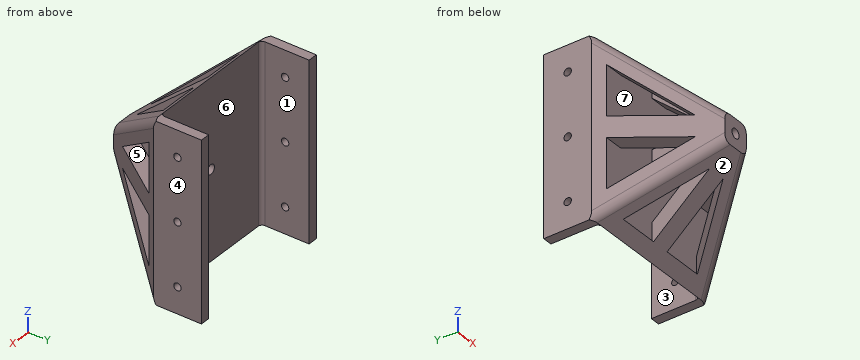
from build123d import *

# Parameters (mm, degrees)
BOSS_EXTRUDE1_DEPTH = 117.094
SKETCH3_R           = 2.4384
CUT_EXTRUDE1_DEPTH  = 166.226170252
SKETCH4_R           = 3.175
CUT_EXTRUDE2_DEPTH  = 166.226170252
CUT_EXTRUDE3_DEPTH  = 166.226170252
FILLET1_R           = 6.35
CUT_EXTRUDE4_DEPTH  = 166.226170252
CUT_EXTRUDE5_DEPTH  = 110.744


with BuildPart() as part:
    # Sketch2 → Boss-Extrude1 (new body)
    with BuildSketch(Plane.XY):
        with BuildLine():
            Line((95.25, 31.75), (101.6, 31.75))
            Line((101.6, 31.75), (101.6, 0))
            Line((101.6, 0), (60.325, -57.15))
            Line((60.325, -57.15), (41.275, -57.15))
            Line((41.275, -57.15), (0, 0))
            Line((0, 0), (0, 31.75))
            Line((0, 31.75), (6.35, 31.75))
            Line((6.35, 31.75), (6.35, 2.54))
            ThreePointArc((6.35, 2.54), (7.093948776, 0.743948776), (8.89, 0))
            Line((8.89, 0), (92.71, 0))
            ThreePointArc((92.71, 0), (94.506051224, 0.743948776), (95.25, 2.54))
            Line((95.25, 2.54), (95.25, 31.75))
        make_face()
    extrude(amount=BOSS_EXTRUDE1_DEPTH)

    # Sketch3 → Cut-Extrude1 (cut, through all)
    with BuildSketch(Plane(origin=(101.6, 0, 0), x_dir=(0, 0, -1), z_dir=(1, 0, 0))):
        with Locations((-99.822, 15.875)):
            Circle(SKETCH3_R)
        with Locations((-58.547, 15.875)):
            Circle(SKETCH3_R)
        with Locations((-17.272, 15.875)):
            Circle(SKETCH3_R)
    extrude(amount=-CUT_EXTRUDE1_DEPTH, mode=Mode.SUBTRACT)

    # Sketch4 → Cut-Extrude2 (cut, through all)
    with BuildSketch(Plane(origin=(0, 0, 0), x_dir=(1, 0, 0), z_dir=(0, 1, 0))):
        with Locations(Location((50.8, -58.547, 0), (0, 0, 270))):
            Circle(SKETCH4_R)
    extrude(amount=-CUT_EXTRUDE2_DEPTH, mode=Mode.SUBTRACT)

    # Sketch5 → Cut-Extrude3 (cut, through all)
    with BuildSketch(Plane(origin=(101.6, 0, 0), x_dir=(0, 0, -1), z_dir=(1, 0, 0))):
        Polygon((-117.094, 0), (-117.094, -57.15), (-68.072, -57.15), align=None)
        Polygon((-49.022, -57.15), (0, -57.15), (0, 0), align=None)
    extrude(amount=-CUT_EXTRUDE3_DEPTH, mode=Mode.SUBTRACT)

    # Fillet1
    fillet1_edges = [part.edges().sort_by_distance(p)[0] for p in [
        (80.9625, -28.575, 92.583),
        (20.6375, -28.575, 92.583),
        (80.9625, -28.575, 24.511),
        (20.6375, -28.575, 24.511),
    ]]
    fillet(fillet1_edges, radius=FILLET1_R)

    # Sketch7 → Cut-Extrude4 (cut, through all)
    with BuildSketch(Plane(origin=(101.6, 0, 0), x_dir=(0, 0, -1), z_dir=(1, 0, 0))):
        Polygon((-98.104076531, -6.35), (-65.422743198, -44.45), (-65.422743198, -6.35), align=None)
        Polygon((-18.989923469, -6.35), (-51.671256802, -6.35), (-51.671256802, -44.45), align=None)
    extrude(amount=-CUT_EXTRUDE4_DEPTH, mode=Mode.SUBTRACT)

    # Sketch8 → Cut-Extrude5 (cut)
    with BuildSketch(Plane.XY.offset(117.094)):
        Polygon((17.266111361, -6.35), (44.782778028, -44.45), (44.782778028, -6.35), align=None)
        Polygon((84.333888639, -6.35), (56.817221972, -6.35), (56.817221972, -44.45), align=None)
    extrude(amount=-CUT_EXTRUDE5_DEPTH, mode=Mode.SUBTRACT)


solid = part.part
Part model, mm, in its own coordinate system. Face numbers are marked on the shaded views. A direction names the side the tool comes from. Coordinates: 2 decimals unless noted, no trailing zeros. Write each loop counter-clockwise with the first axis right and the second up, starting at its lowest first coordinate (ties: lowest second). Pieces come first, ordered by that corner, then holes. Notation, with made-up numbers: (-2, -29) - (44, -29) arc R13 cw to (44, -15) - close; hole circle Ø10 at (34.25, 56.25). An arc over 180 degrees is marked (long way). Put each result on its own line as item: value.
1. 3-axis set-ups, long thin cutter, end or side, ignore diameter. For the marked faces 5, 6 and 7: which of +Z, -Z, +X, -X, +Y, -Y reach the whole face in a straight line?
Final values:
face 5: +X, -X
face 6: +Z, -Z, +Y
face 7: none
2. Two-plate mould, pull along X, no slides. Class the marked faces 1, 2, 3 and 4: +X half, -X half, draft (parallel to the pull), parting line (faces both ways), or undercut.
Final values:
face 1: undercut
face 2: draft
face 3: undercut
face 4: +X half
3. Probe line 1 along X through (y, z) = (12, 25.5); line 2 along Z through (x, y) = (50.5, -39); line 3 along X through (y, z) = (-36, 41.5). List the from-to ranges inside material, lowest first. Write a range as [from, to].
Final values:
line 1: x = [0, 6.35], [95.25, 101.6]
line 2: z = [33.45, 47], [51.67, 55.39], [61.71, 65.42], [70.1, 83.64]
line 3: x = [26, 38.68], [44.78, 56.82], [62.92, 75.6]
4. Band-saw the part on B-B (x = 50.8). Write the cut outline in (y, z).
Final values:
outline: (-57.15, 49.02) - (0, 0) - (0, 55.37) - (-57.15, 55.37) - close; (-57.15, 61.72) - (0, 61.72) - (0, 117.09) - (-57.15, 68.07) - close; hole (-44.45, 51.67) - (-6.35, 18.99) - (-6.35, 51.67) - close; hole (-44.45, 65.42) - (-6.35, 65.42) - (-6.35, 98.1) - close
5. Band-saw the part on C-C (z = 27). Give the number of separate pieces and of enclosed holes in the cut face, then the cut area to 3 significant figures.
Final values:
separate pieces: 4
enclosed holes: 0
area: 1,600 mm²
6. Flat gauge pins, fed straight in: pin 1 Ø4 at (y, z) = (15.875, 17.272) entering from +X; pin 2 Ø11.5 at (y, z) = (-17.5, 24.5) entering from +X; pin 3 Ø5 at (x, z) = (30, 46.5) entering from +Y; pin 4 Ø9.5 at (x, y) = (51, -28) entering from -Z. Where does each tip first touch, or does it go through?
Final values:
pin 1: passes through
pin 2: stops at x = 93.07
pin 3: stops at y = 0
pin 4: stops at z = 19.94
7. Band-saw the part on A-A (y = 5). Write the cut outline in (x, z), then the cut area to 3 significant figures.
Final values:
outline: (0, 0) - (6.35, 0) - (6.35, 117.09) - (0, 117.09) - close; (95.25, 0) - (101.6, 0) - (101.6, 117.09) - (95.25, 117.09) - close
area: 1,490 mm²
